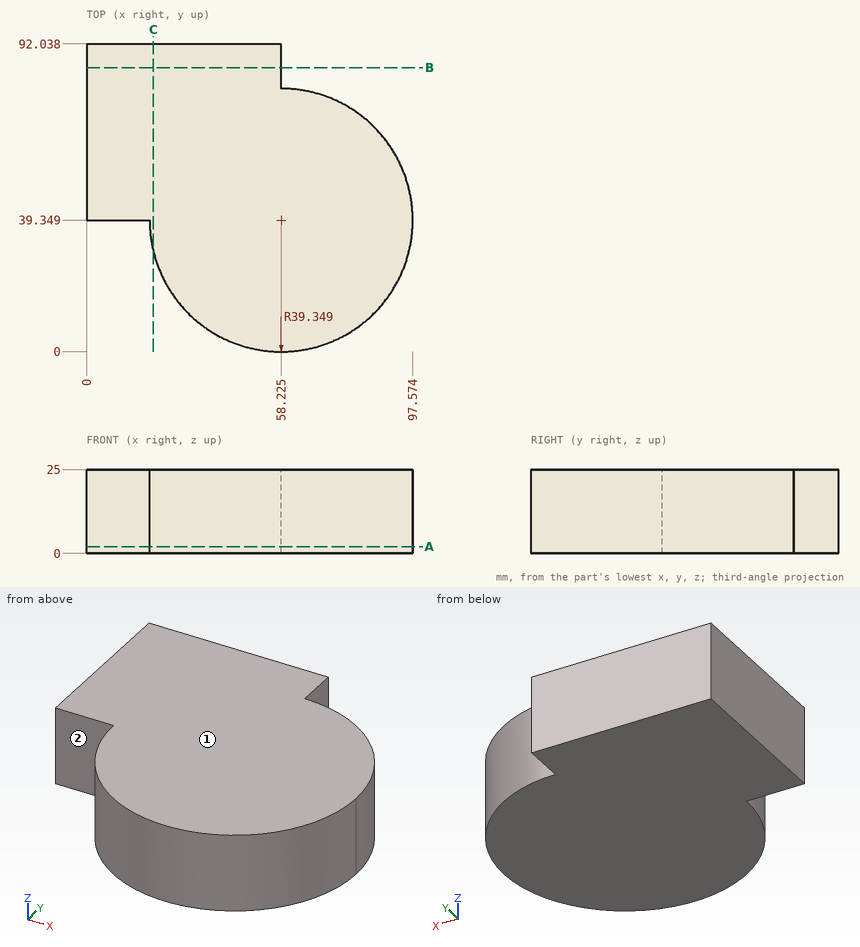
Verification items for this drawing (mm, ordinates from the low corner). A direction names the side the tool comes from. Round coordinates to 2 decimals unless told otherwise and drop trailing zeros. Order: outer loops, then holes, each group sorted by start corner. A loop starts at its lowest first (then second) coordinate and runs counter-clockwise, first axis right, second up. Notation, with made-up numbers: M 6,-35 L 53,-35 A9 ccw 53,-18 Z; hole C -14.75,64 d1. An arc over 180 degrees is marked long. Answer in a Markdown table with one row per item. Add a question column.
Item 1: Sectioned sample at C-C, the plane x = 20. Enter the section's corners in (y, z).
Item 2: Sectioned sample at A-A, the plane z = 2. Enter the section's corners in (x, y) (1 decimal).
Item 3: Set-up check for the marked faces 1 and 2: record each of +Z, -Z, +X, -X, +Y, -Y from which the full face is reachable in a straight line by a thin tool's end or side.
Item 4: Material ranges on L1, parallel to X at y = 40, z = 19; L2, parallel to Y at x = 18.5, z = 4; L3, parallel to X at y = 6.5, z = 15.5 (1 decimal), recorded low to high. Write a range as [from, to].
Item 5: Depth check by flat-ended pin: pin 1 Ø1.5 at (y, z) = (36.5, 17) entering from -X; pin 2 Ø6 at (y, z) = (27, 7) entering from -X; pin 3 Ø6 at (y, z) = (23.5, 15) entering from +X. Enter the tip coordinate at first touch or a pass-through.
Item 6: Sectioned sample at B-B, the plane y = 85. Enter the section's corners in (x, z) (1 decimal), plus the area to 3 significant figures.
Filled in:
| question | item | result |
|---|---|---|
| 1 | outline | M 30.01,0 L 92.04,0 L 92.04,25 L 30.01,25 Z |
| 2 | outline | M 0,39.3 L 18.9,39.3 A39.3 ccw long 58.2,78.7 L 58.2,92 L 0,92 Z |
| 3 | face 1 | +Z, +X, -X, +Y, -Y |
| 3 | face 2 | +Z, -Z, -X, -Y |
| 4 | L1 | x = [0, 97.57] |
| 4 | L2 | y = [39.35, 92.04] |
| 4 | L3 | x = [36.6, 79.9] |
| 5 | pin 1 | stops at x = 18.93 |
| 5 | pin 2 | stops at x = 20 |
| 5 | pin 3 | stops at x = 95.42 |
| 6 | outline | M 0,0 L 58.2,0 L 58.2,25 L 0,25 Z |
| 6 | area | 1,460 mm² |
